Source: CAD feature listing. Evaluate the final solid. Frame: model axes, mm. A direction names the side the tool comes from. Round coordinates to 2 decimals unless told otherwise and drop trailing zeros. Order: outer loops, then holes, each group sorted by start corner. A loop starts at its lowest first (then second) coordinate and runs counter-clockwise, first axis right, second up. Notation, with made-up numbers: (-5.5, 58) - (0.5, 58) arc R33 cw to (0.5, 92) - close; hole circle Ø8 at (-22.75, 81.5). An arc over 180 degrees is marked (long way). Return JSON: item names as keys, results as strings. Group by question number.
1) Access query for faces 1 (the flat face through (-2, -20, 1)), 2 (the flat face through (135, -69, -1)). Directions: +Z, -Z, +X, -X, +Y, -Y. A direction counts if a zero-diameter tool reaches every point of the face in a straight line with its end or side. Return the directions, or none.
2) Section A-A, the plane y = -57.5. Return loops of the section in (x, z), plus the area to 3 significant figures.
3) Section B-B, the plane x = -80. Return loops of the section in (y, z).
4) Section C-C, the plane z = 30. Return loops of the section in (x, y).
5) Ray query, line 1 (Z direction, x = -79, y = -78.5); line 2 (X direction, y = -50, z = 26.5); line 3 (Y direction, x = 39, z = 39.5). Return the intervals inside material, ascending. Write a range as from..to.
6) Contact query for a flat-ended pin moving along its axis: P1, Ø6, axis at x = 60.5, z = -32, coming from the +Y side. Output: stop coordinate, or through.
```python
from build123d import *

# Parameters (mm, degrees)
F0_W     = 270
F0_H     = 140
F1_DEPTH = 140
F2_W     = 250
F2_H     = 120
F3_DEPTH = 120
F4_R     = 20


with BuildPart() as f1:
    # F0 (on Front) → F1 (new body)
    with BuildSketch(Plane.XZ):
        Rectangle(F0_W, F0_H)
    extrude(amount=F1_DEPTH)

    # F2 (on face) → F3 (cut)
    with BuildSketch(Plane.XZ.offset(140)):
        Rectangle(F2_W, F2_H)
    extrude(amount=-F3_DEPTH, mode=Mode.SUBTRACT)

    # F4
    f4_edges = [f1.edges().sort_by_distance(p)[0] for p in [
        (135, -70, 70),
        (-135, -70, 70),
        (135, -70, -70),
        (-135, -70, -70),
    ]]
    fillet(f4_edges, radius=F4_R)


solid = f1.part
```
Geometry check:
{
 "1": {"face 1": "-Y", "face 2": "+Z, -Z, +X, +Y, -Y"},
 "2": {"outline": "(-135, -50) arc R20 ccw to (-115, -70) - (115, -70) arc R20 ccw to (135, -50) - (135, 50) arc R20 ccw to (115, 70) - (-115, 70) arc R20 ccw to (-135, 50) - close; hole (-125, -60) - (125, -60) - (125, 60) - (-125, 60) - close", "area": "7,460 mm2"},
 "3": {"outline": "(-140, -70) - (0, -70) - (0, 70) - (-140, 70) - (-140, 60) - (-20, 60) - (-20, -60) - (-140, -60) - close"},
 "4": {"outline": "(-135, -140) - (-125, -140) - (-125, -20) - (125, -20) - (125, -140) - (135, -140) - (135, 0) - (-135, 0) - close"},
 "5": {"line 1": "-70..-60, 60..70", "line 2": "-135..-125, 125..135", "line 3": "-20..0"},
 "6": {"P1": "y = 0"}
}
